Autodesk Inventor part; units mm, degrees
ref_plane "YZ Plane" through (0, 0, 0) normal (1, 0, 0) x (0, 1, 0)
ref_plane "XZ Plane" through (0, 0, 0) normal (0, 1, 0) x (-1, 0, 0)
ref_plane "XY Plane" through (0, 0, 0) normal (0, 0, 1) x (1, 0, 0)
sketch "Sketch1" plane through (0, 0, 0) normal (0, 0, 1) x (1, 0, 0)
  line L0 (0, 0) -> (152.4, 0)
  line L1 (152.4, 0) -> (152.4, 152.4)
  line L2 (152.4, 152.4) -> (0, 152.4)
  line L3 (0, 152.4) -> (0, 0)
  dimension "d0" = 152.4
  dimension "d1" = 152.4
extrude "Extrusion1" add sketch "Sketch1" along normal blind 152.4
sketch "Sketch2" plane through (0, 0, 152.4) normal (0, 0, 1) x (1, 0, 0)
  line L0 (50.8, 50.8) -> (101.6, 50.8)
  line L1 (101.6, 50.8) -> (101.6, 101.6)
  line L2 (101.6, 101.6) -> (50.8, 101.6)
  line L3 (50.8, 101.6) -> (50.8, 50.8)
  line L4 (152.4, 152.4) -> (0, 152.4)
  line L5 (152.4, 0) -> (152.4, 152.4)
  point P0 (0, 0)
  dimension "d4" = 50.8
  dimension "d5" = 50.8
  dimension "d6" = 50.8
  dimension "d7" = 50.8
extrude "Extrusion2" cut sketch "Sketch2" against normal blind 182.5625
sketch "Sketch3" plane through (152.4, 0, 0) normal (1, 0, 0) x (0, 0, -1)
  line L0 (-101.6, 50.8) -> (-50.8, 50.8)
  line L1 (-50.8, 50.8) -> (-50.8, 101.6)
  line L2 (-50.8, 101.6) -> (-101.6, 101.6)
  line L3 (-101.6, 101.6) -> (-101.6, 50.8)
  line L4 (0, 152.4) -> (-152.4, 152.4)
  line L5 (-152.4, 0) -> (-152.4, 152.4)
  point P0 (0, 0)
  dimension "d10" = 50.8
  dimension "d11" = 50.8
  dimension "d12" = 50.8
  dimension "d13" = 50.8
extrude "Extrusion3" cut sketch "Sketch3" against normal blind 182.5625
sketch "Sketch4" plane through (0, 152.4, 0) normal (0, 1, 0) x (1, 0, 0)
  line L0 (101.6, -101.6) -> (50.8, -101.6)
  line L1 (50.8, -101.6) -> (50.8, -50.8)
  line L2 (50.8, -50.8) -> (101.6, -50.8)
  line L3 (101.6, -50.8) -> (101.6, -101.6)
  line L4 (152.4, -152.4) -> (0, -152.4)
  line L5 (0, 0) -> (0, -152.4)
  dimension "d16" = 50.8
  dimension "d17" = 50.8
  dimension "d18" = 50.8
  dimension "d19" = 50.8
extrude "Extrusion4" cut sketch "Sketch4" against normal blind 182.5625
fillet "Fillet1" radius 12.7 12 edges at (76.2, 152.4, 152.4) (152.4, 152.4, 76.2) (0, 76.2, 152.4) (76.2, 0, 152.4) (152.4, 0, 76.2) (152.4, 76.2, 152.4) (152.4, 76.2, 0) (0, 152.4, 76.2) (76.2, 152.4, 0) (0, 0, 76.2) (0, 76.2, 0) (76.2, 0, 0)
properties part number "cube practice"
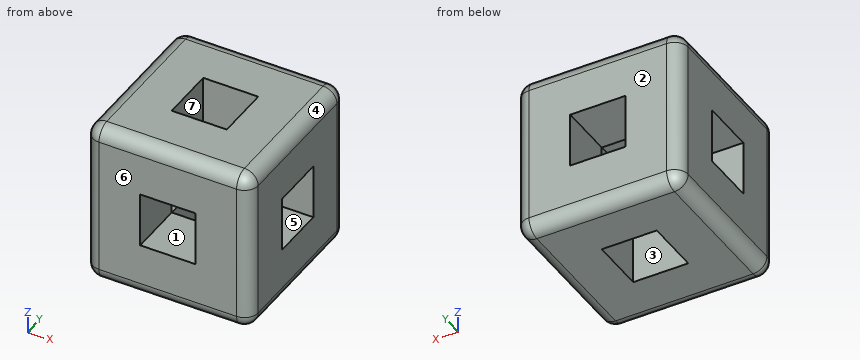
Check sheet for the modelled part. Datum: model origin and axes. Units: mm. Face numbers are marked on the shaded views. A direction names the side the tool comes from. Coordinates: 2 decimals unless noted, no trailing zeros. Order: outer loops, then holes, each group sorted by start corner. A loop starts at its lowest first (then second) coordinate and runs counter-clockwise, first axis right, second up. Notation, with made-up numbers: M 64,39.25 L 105,39.25 A8 ccw 105,51.25 Z; hole C -5,41 d1. An arc over 180 degrees is marked long. Write each question's results on one line, items separated by ' | '. Start each with the question number.
1. Material ranges on probe 1 along Y at (x, z) = (85, 129.5), recorded low to high.
2. Cross-section at B-B on z = 134.5. Record the cut outline in (x, y).
3. Access from +Z, -Z, +X, -X, +Y, -Y to the whole of each face (thin tool, end or side, straight path). Record for the marked faces 5, 6 and 7.
4. Cross-section at A-A on x = 57. Record the cut outline in (y, z).
5. Mould release check, pull along X, two halves, no side actions. Record for the marked faces 1, 2, 3 and 4: +X half, -X half, draft (parallel to the pull), parting line (faces both ways), or undercut.
Checks:
1) probe 1: y = 0 to 50.8, 101.6 to 152.4
2) outline: M 0,12.7 A12.7 ccw 12.7,0 L 139.7,0 A12.7 ccw 152.4,12.7 L 152.4,139.7 A12.7 ccw 139.7,152.4 L 12.7,152.4 A12.7 ccw 0,139.7 Z; hole M 50.8,50.8 L 101.6,50.8 L 101.6,101.6 L 50.8,101.6 Z
3) face 5: +X, -X | face 6: +Z, -Z, +X, -X, -Y | face 7: +Z, -Z
4) outline: M 0,12.7 A12.7 ccw 12.7,0 L 50.8,0 L 50.8,50.8 L 0,50.8 Z; M 0,101.6 L 50.8,101.6 L 50.8,152.4 L 12.7,152.4 A12.7 ccw 0,139.7 Z; M 101.6,0 L 139.7,0 A12.7 ccw 152.4,12.7 L 152.4,50.8 L 101.6,50.8 Z; M 101.6,101.6 L 152.4,101.6 L 152.4,139.7 A12.7 ccw 139.7,152.4 L 101.6,152.4 Z
5) face 1: undercut | face 2: draft | face 3: undercut | face 4: +X half
